Autodesk Inventor part; units mm, degrees
ref_plane "YZ Plane" through (0, 0, 0) normal (1, 0, 0) x (0, 1, 0)
ref_plane "XZ Plane" through (0, 0, 0) normal (0, 1, 0) x (-1, 0, 0)
ref_plane "XY Plane" through (0, 0, 0) normal (0, 0, 1) x (1, 0, 0)
sketch "Sketch1" plane through (0, 0, 0) normal (1, 0, 0) x (0, 1, 0)
  circle A0 centre (0, 0) radius 5.5563
  dimension "d0" = 11.1125
extrude "Extrusion1" add sketch "Sketch1" along normal blind 76.2
chamfer "Chamfer1" distance 0.762 angle 45 2 edges at (76.2, -5.5563, 0) (0, -5.5563, 0)
sketch "Sketch2" plane through (76.2, 0, 0) normal (1, 0, 0) x (0, 0, -1)
  point P0 (0, 0)
sketch "Sketch3" plane through (76.2, 0, 0) normal (1, 0, 0) x (0, 0, -1)
  point P0 (0, 0)
  point P1 (0, 0)
hole "Hole1" at (76.2, 0, 0) direction (-1, 0, 0) diameter 4.9784 depth 19.05 tip angle 118
sketch "Sketch4" plane through (0, 0, 0) normal (-1, 0, 0) x (0, 0, 1)
  point P0 (0, 0)
ref_plane "Work Plane2" through (4.7625, 0, 0) normal (-1, 0, 0) x (0, 0, 1)
sketch "Sketch5" plane through (4.7625, 0, 0) normal (-1, 0, 0) x (0, 0, 1)
  circle A0 centre (0, 0) radius 5.5562
  circle A1 centre (0, 0) radius 4.2344
extrude "Extrusion2" cut sketch "Sketch5" against normal blind 1.5875
properties part number "upper die center pin"
Model file for the job. Use its own axes, mm. A direction names the side the tool comes from. Round coordinates to 2 decimals unless told otherwise and drop trailing zeros. Order: outer loops, then holes, each group sorted by start corner. A loop starts at its lowest first (then second) coordinate and runs counter-clockwise, first axis right, second up.
(1) 3-axis set-ups, long thin cutter, end or side, ignore diameter. For faces 4 (the face through (4.762, -2, -4)), 5 (the face through (40.41, -1.204, 5.424)): which of +Z, -Z, +X, -X, +Y, -Y reach the whole face in a straight line?
(2) Pin check, flat tips, straight feed: pin 1 (1.5 mm diameter, centred on x = 50, y = 2, fed in from +Z); pin 2 (2 mm diameter, centred on x = 29, y = -2, fed in from -Z); pin 3 (6 mm diameter, centred on x = 13.5, y = 3.5, fed in from +Z). Stop position of each tip, or through.
(3) Drill centre lines: line 1 (Z direction, x = 71.5, y = 0); line 2 (X direction, y = 2.75, z = 3.75). Where is each one in solid material? Low to high.
(4) Band-saw the part on A-A (x = 18). List the corners of the cut face in (y, z).
(5) Pull direction Y, two halves, no side cores. Call faces 1 (the face through (66.542, -0.748, -2.374)), 2 (the face through (5.55, -2.58, -3.36)), 3 (the face through (0, 0, 0)): released by +Y, released by -Y, zero draft, split by the parting line, or undercut.
Verdict:
1. face 4: none
1. face 5: +X, -X
2. pin 1: stops at z = 5.41
2. pin 2: stops at z = -5.47
2. pin 3: stops at z = 5.53
3. line 1: z = -5.56 to -2.49, 2.49 to 5.56
3. line 2: x = 0 to 4.76, 6.35 to 76.2
4. outline: circle Ø11.11 at (0, 0)
5. face 1: undercut
5. face 2: split by the parting line
5. face 3: zero draft
